Design review of the part built by this model. Coordinates are the model's own, in mm. A direction names the side the tool comes from. Coordinates: 2 decimals unless noted, no trailing zeros. Write each loop counter-clockwise with the first axis right and the second up, starting at its lowest first coordinate (ties: lowest second). Pieces come first, ordered by that corner, then holes. Notation, with made-up numbers: (-35, 7) - (-18, 7) arc R31 cw to (-18, 31) - close; hole circle Ø9 at (17, -31). An arc over 180 degrees is marked (long way). Answer as a JSON object with one key per item and string values.
```python
from build123d import *

# Parameters (mm, degrees)
SKETCH_R      = 11
PAD_DEPTH     = 0.3
SKETCH001_R   = 11
SKETCH001_R_2 = 10.2
PAD001_DEPTH  = 10
CHAMFER_SIZE  = 0.6


with BuildPart() as part:
    # Sketch → Pad (new body)
    with BuildSketch(Plane.XY):
        Circle(SKETCH_R)
    extrude(amount=PAD_DEPTH)

    # Sketch001 (on Face3 of Pad) → Pad001 (join)
    with BuildSketch(Plane.XY.offset(0.3)):
        Circle(SKETCH001_R)
        Circle(SKETCH001_R_2, mode=Mode.SUBTRACT)
    extrude(amount=PAD001_DEPTH)

    # Chamfer
    chamfer_edges = [part.edges().sort_by_distance(p)[0] for p in [
        (-11, 0, 10.3),
    ]]
    chamfer(chamfer_edges, length=CHAMFER_SIZE)


solid = part.part
```
(1) Take a section at C-C, the plane z = 5.5. Write out the cut boundary in (x, y).
Solved:
{"outline": "circle Ø22 at (0, 0); hole circle Ø20.4 at (0, 0)"}
(2) Take a section at A-A, the plane x = 0. Write out the cut boundary in (y, z).
Solved:
{"outline": "(-11, 0) - (11, 0) - (11, 9.7) - (10.4, 10.3) - (10.2, 10.3) - (10.2, 0.3) - (-10.2, 0.3) - (-10.2, 10.3) - (-10.4, 10.3) - (-11, 9.7) - close"}
(3) To check wall thickness, follow line 1 (Y direction, x = 0, z = 7); line 2 (Z direction, x = 0.25, y = 9.5); line 3 (Y direction, x = -2.25, z = 3). State the ranges of each line that lie inside material, in increasing order. Write a range as from..to.
Solved:
{"line 1": "y = -11..-10.2, 10.2..11", "line 2": "z = 0..0.3", "line 3": "y = -10.77..-9.95, 9.95..10.77"}
(4) Tool access review of faces 1 (the face through (4.707, -9.049, 5.23)), 2 (the face through (0, 0, 0)): name each direction out of +Z, -Z, +X, -X, +Y, -Y from which nothing blocks a thin tool from reaching the whole face with its end or side.
Solved:
{"face 1": "+Z", "face 2": "-Z, +X, -X, +Y, -Y"}
(5) For pin 1 (3 mm diameter, centred on y = -0.5, z = 6.5, fed in from +X); pin 2 (6 mm diameter, centred on x = -5.5, z = 5, fed in from +Y); pin 3 (6 mm diameter, centred on x = -5, z = 7, fed in from +Y); pin 4 (6 mm diameter, centred on x = -3, y = 4, fed in from +Z), all flat-tipped, find the tip position at first contact; note any pin that passes through.
Solved:
{"pin 1": "stops at x = 11", "pin 2": "stops at y = 10.71", "pin 3": "stops at y = 10.82", "pin 4": "stops at z = 0.3"}
